```python
from build123d import *

# Parameters (mm, degrees)
BOX_W                  = 7.4
BOX_H                  = 7
BOX_DEPTH              = 0.2
BOX015_W               = 0.8
BOX015_H               = 9.4
BOX015_DEPTH           = 0.8
BOX015_PLACEMENT_ANGLE = 225
BOX014_W               = 0.4
BOX014_H               = 2.3
BOX014_DEPTH           = 1.91
BOX017_W               = 0.8
BOX017_H               = 9.4
BOX017_DEPTH           = 0.8
BOX017_PLACEMENT_ANGLE = 45
BOX013_W               = 0.4
BOX013_H               = 2.3
BOX013_DEPTH           = 1.91
BOX018_W               = 7.4
BOX018_H               = 9.4
BOX018_DEPTH           = 3.7
CYLINDER004_R          = 0.25
CYLINDER004_DEPTH      = 0.17
BOX024_W               = 0.9
BOX024_H               = 1.5
BOX024_DEPTH           = 0.15
FILLET006_R            = 0.2
CYLINDER006_R          = 0.25
CYLINDER006_DEPTH      = 0.17
BOX025_W               = 0.9
BOX025_H               = 1.5
BOX025_DEPTH           = 0.15
FILLET007_R            = 0.2
CYLINDER005_R          = 0.25
CYLINDER005_DEPTH      = 0.17
BOX026_W               = 0.9
BOX026_H               = 1.5
BOX026_DEPTH           = 0.15
FILLET008_R            = 0.2
CYLINDER007_R          = 0.25
CYLINDER007_DEPTH      = 0.17
BOX027_W               = 0.9
BOX027_H               = 1.5
BOX027_DEPTH           = 0.15
FILLET005_R            = 0.2
BOX023_W               = 0.8
BOX023_H               = 2.2
BOX023_DEPTH           = 0.8
BOX023_PLACEMENT_ANGLE = 45
BOX022_W               = 0.4
BOX022_H               = 2.2
BOX022_DEPTH           = 2
BOX020_W               = 0.8
BOX020_H               = 2.2
BOX020_DEPTH           = 0.8
BOX020_PLACEMENT_ANGLE = 45
BOX021_W               = 0.4
BOX021_H               = 2.2
BOX021_DEPTH           = 2
BOX019_W               = 7.7
BOX019_H               = 9.2
BOX019_DEPTH           = 4
FILLET009_R            = 0.2


with BuildPart() as cube:
    # Box → Box (new body)
    with BuildSketch(Plane(origin=(0.15, 2.2, -0.01), x_dir=(1, 0, 0), z_dir=(0, 0, 1))):
        with Locations((3.7, 3.5)):
            Rectangle(BOX_W, BOX_H)
    extrude(amount=BOX_DEPTH)


with BuildPart() as cube011:
    # Box015 → Box015 (new body)
    with BuildSketch(Plane.XY):
        with Locations((0.4, 4.7)):
            Rectangle(BOX015_W, BOX015_H)
    extrude(amount=BOX015_DEPTH)


with BuildPart() as cube011_1:
    # Box015 placement: moved
    add(cube011.part.moved(Location((7.4, -0.1, 2.06))).rotate(Axis((7.4, -0.1, 2.06), (0, 1, 0)), BOX015_PLACEMENT_ANGLE))


with BuildPart() as cut013:
    # Box014 → Box014 (new body)
    with BuildSketch(Plane(origin=(7, -0.1, 0.15), x_dir=(1, 0, 0), z_dir=(0, 0, 1))):
        with Locations((0.2, 1.15)):
            Rectangle(BOX014_W, BOX014_H)
    extrude(amount=BOX014_DEPTH)

    # Cut013: cut Cube011
    add(cube011_1.part, mode=Mode.SUBTRACT)


with BuildPart() as cut013_1:
    # Cut013 placement: moved
    add(cut013.part.moved(Location((0.15, 0, 0))))


with BuildPart() as cube013:
    # Box017 → Box017 (new body)
    with BuildSketch(Plane.XY):
        with Locations((0.4, 4.7)):
            Rectangle(BOX017_W, BOX017_H)
    extrude(amount=BOX017_DEPTH)


with BuildPart() as cube013_1:
    # Box017 placement: moved
    add(cube013.part.moved(Location((0.15, -0.1, 2.06))).rotate(Axis((0.15, -0.1, 2.06), (0, 1, 0)), BOX017_PLACEMENT_ANGLE))


with BuildPart() as cut022:
    # Box013 → Box013 (new body)
    with BuildSketch(Plane(origin=(0.15, -0.1, 0.15), x_dir=(1, 0, 0), z_dir=(0, 0, 1))):
        with Locations((0.2, 1.15)):
            Rectangle(BOX013_W, BOX013_H)
    extrude(amount=BOX013_DEPTH)

    # Cut022: cut Cube013
    add(cube013_1.part, mode=Mode.SUBTRACT)


with BuildPart() as cut024:
    # Box018 → Box018 (new body)
    with BuildSketch(Plane(origin=(0.15, -0.1, 0.15), x_dir=(1, 0, 0), z_dir=(0, 0, 1))):
        with Locations((3.7, 4.7)):
            Rectangle(BOX018_W, BOX018_H)
    extrude(amount=BOX018_DEPTH)

    # Cut023: cut Cut022
    add(cut022.part, mode=Mode.SUBTRACT)

    # Cut024: cut Cut013
    add(cut013_1.part, mode=Mode.SUBTRACT)


with BuildPart() as cylinder004:
    # Cylinder004 → Cylinder004 (new body)
    with BuildSketch(Plane(origin=(-0.9, 2.95, -0.01), x_dir=(1, 0, 0), z_dir=(0, 0, 1))):
        Circle(CYLINDER004_R)
    extrude(amount=CYLINDER004_DEPTH)


with BuildPart() as foot012:
    # Box024 → Box024 (new body)
    with BuildSketch(Plane(origin=(-0.9, 2.2, 0), x_dir=(1, 0, 0), z_dir=(0, 0, 1))):
        with Locations((0.45, 0.75)):
            Rectangle(BOX024_W, BOX024_H)
    extrude(amount=BOX024_DEPTH)

    # Cut021: cut Cylinder004
    add(cylinder004.part, mode=Mode.SUBTRACT)

    # Fillet006
    fillet006_edges = [foot012.edges().sort_by_distance(p)[0] for p in [
        (-0.9, 2.7, 0.075),
        (-0.9, 2.2, 0.075),
        (-0.9, 3.2, 0.075),
        (-0.9, 3.7, 0.075),
    ]]
    fillet(fillet006_edges, radius=FILLET006_R)


with BuildPart() as cylinder006:
    # Cylinder006 → Cylinder006 (new body)
    with BuildSketch(Plane(origin=(-0.9, 8.45, -0.01), x_dir=(1, 0, 0), z_dir=(0, 0, 1))):
        Circle(CYLINDER006_R)
    extrude(amount=CYLINDER006_DEPTH)


with BuildPart() as foot013:
    # Box025 → Box025 (new body)
    with BuildSketch(Plane(origin=(-0.9, 7.7, 0), x_dir=(1, 0, 0), z_dir=(0, 0, 1))):
        with Locations((0.45, 0.75)):
            Rectangle(BOX025_W, BOX025_H)
    extrude(amount=BOX025_DEPTH)

    # Cut016: cut Cylinder006
    add(cylinder006.part, mode=Mode.SUBTRACT)

    # Fillet007
    fillet007_edges = [foot013.edges().sort_by_distance(p)[0] for p in [
        (-0.9, 8.2, 0.075),
        (-0.9, 7.7, 0.075),
        (-0.9, 8.7, 0.075),
        (-0.9, 9.2, 0.075),
    ]]
    fillet(fillet007_edges, radius=FILLET007_R)


with BuildPart() as cylinder005:
    # Cylinder005 → Cylinder005 (new body)
    with BuildSketch(Plane(origin=(8.6, 2.95, -0.01), x_dir=(1, 0, 0), z_dir=(0, 0, 1))):
        Circle(CYLINDER005_R)
    extrude(amount=CYLINDER005_DEPTH)


with BuildPart() as foot014:
    # Box026 → Box026 (new body)
    with BuildSketch(Plane(origin=(7.7, 2.2, 0), x_dir=(1, 0, 0), z_dir=(0, 0, 1))):
        with Locations((0.45, 0.75)):
            Rectangle(BOX026_W, BOX026_H)
    extrude(amount=BOX026_DEPTH)

    # Cut014: cut Cylinder005
    add(cylinder005.part, mode=Mode.SUBTRACT)

    # Fillet008
    fillet008_edges = [foot014.edges().sort_by_distance(p)[0] for p in [
        (8.6, 2.2, 0.075),
        (8.6, 3.7, 0.075),
        (8.6, 2.7, 0.075),
        (8.6, 3.2, 0.075),
    ]]
    fillet(fillet008_edges, radius=FILLET008_R)


with BuildPart() as cylinder007:
    # Cylinder007 → Cylinder007 (new body)
    with BuildSketch(Plane(origin=(8.6, 8.45, -0.01), x_dir=(1, 0, 0), z_dir=(0, 0, 1))):
        Circle(CYLINDER007_R)
    extrude(amount=CYLINDER007_DEPTH)


with BuildPart() as foot009:
    # Box027 → Box027 (new body)
    with BuildSketch(Plane(origin=(7.7, 7.7, 0), x_dir=(1, 0, 0), z_dir=(0, 0, 1))):
        with Locations((0.45, 0.75)):
            Rectangle(BOX027_W, BOX027_H)
    extrude(amount=BOX027_DEPTH)

    # Cut015: cut Cylinder007
    add(cylinder007.part, mode=Mode.SUBTRACT)

    # Fillet005
    fillet005_edges = [foot009.edges().sort_by_distance(p)[0] for p in [
        (8.6, 7.7, 0.075),
        (8.6, 9.2, 0.075),
        (8.6, 8.2, 0.075),
        (8.6, 8.7, 0.075),
    ]]
    fillet(fillet005_edges, radius=FILLET005_R)


with BuildPart() as cube019:
    # Box023 → Box023 (new body)
    with BuildSketch(Plane.XY):
        with Locations((0.4, 1.1)):
            Rectangle(BOX023_W, BOX023_H)
    extrude(amount=BOX023_DEPTH)


with BuildPart() as cube019_1:
    # Box023 placement: moved
    add(cube019.part.moved(Location((0, 0, 2))).rotate(Axis((0, 0, 2), (0, 1, 0)), BOX023_PLACEMENT_ANGLE))


with BuildPart() as right_side_cutout001:
    # Box022 → Box022 (new body)
    with BuildSketch(Plane.XY):
        with Locations((0.2, 1.1)):
            Rectangle(BOX022_W, BOX022_H)
    extrude(amount=BOX022_DEPTH)

    # Cut018: cut Cube019
    add(cube019_1.part, mode=Mode.SUBTRACT)


with BuildPart() as right_side_cutout001_1:
    # Cut018 placement: moved
    add(right_side_cutout001.part.moved(Location((7.7, 0, 0))))


with BuildPart() as part_mirroring001:
    # Part__Mirroring001: instance of Right Side Cutout001
    add(right_side_cutout001_1.part.mirror(Plane(origin=(7.7, 0, 0), x_dir=(0, -1, 0), z_dir=(1, 0, 0))))


with BuildPart() as cube016:
    # Box020 → Box020 (new body)
    with BuildSketch(Plane.XY):
        with Locations((0.4, 1.1)):
            Rectangle(BOX020_W, BOX020_H)
    extrude(amount=BOX020_DEPTH)


with BuildPart() as cube016_1:
    # Box020 placement: moved
    add(cube016.part.moved(Location((0, 0, 2))).rotate(Axis((0, 0, 2), (0, 1, 0)), BOX020_PLACEMENT_ANGLE))


with BuildPart() as left_side_cutout001:
    # Box021 → Box021 (new body)
    with BuildSketch(Plane.XY):
        with Locations((0.2, 1.1)):
            Rectangle(BOX021_W, BOX021_H)
    extrude(amount=BOX021_DEPTH)

    # Cut020: cut Cube016
    add(cube016_1.part, mode=Mode.SUBTRACT)


with BuildPart() as metal_shell:
    # Box019 → Box019 (new body)
    with BuildSketch(Plane.XY):
        with Locations((3.85, 4.6)):
            Rectangle(BOX019_W, BOX019_H)
    extrude(amount=BOX019_DEPTH)

    # Cut019: cut Left Side Cutout001
    add(left_side_cutout001.part, mode=Mode.SUBTRACT)

    # Cut017: cut Part__Mirroring001
    add(part_mirroring001.part, mode=Mode.SUBTRACT)

    # Fillet009
    fillet009_edges = [metal_shell.edges().sort_by_distance(p)[0] for p in [
        (0, 4.6, 4),
        (7.7, 4.6, 4),
    ]]
    fillet(fillet009_edges, radius=FILLET009_R)

    # Fusion001: union Foot012, Foot013, Foot014, Foot009
    add(foot012.part)
    add(foot013.part)
    add(foot014.part)
    add(foot009.part)

    # Cut025: cut Cut024
    add(cut024.part, mode=Mode.SUBTRACT)

    # Cut: cut Cube
    add(cube.part, mode=Mode.SUBTRACT)


solid = metal_shell.part
```
Geometry: final body of the model. Coordinates: model frame, mm. Round coordinates to 2 decimals unless told otherwise and drop trailing zeros. Write each loop counter-clockwise with the first axis right and the second up, starting at its lowest first coordinate (ties: lowest second). Pieces come first, ordered by that corner, then holes. Notation, with made-up numbers: M -30.5,12.25 L -7.5,12.25 A9 cw -7.5,28.25 Z; hole C -29,75 d5. An arc over 180 degrees is marked long. Answer in a Markdown table with one row per item. Add a question column.
(1) Cut plane C-C, the plane z = 3.4. Return the cut outline in (x, y).
(2) Cut plane D-D, the plane y = 1.25. Return the cut outline in (x, z).
(3) Draft query along Z for faces 1 (the face through (0.55, 1, 1)), 2 (the face through (0.4, 1, 1)). Return one class per face: pulls with the +Z half, pulls with the -Z half, needs draft (parallel to the pull), parting line crosses it, or undercut.
(4) Ray query, L1, parallel to X at y = 1, z = 0.95. Return the intervals inside material, ascending.
(5) Contact query for flat-ended pins moving along their axis: pin 1 (1 mm diameter, centred on y = 6, z = 3.5, fed in from -X); pin 2 (0.7 mm diameter, centred on x = 8.5, y = 2.5, fed in from +Z); pin 3 (1 mm diameter, centred on x = 1, z = 1, fed in from +Y); pin 4 (0.7 mm diameter, centred on x = -0.5, z = 1.5, fed in from -Y). Output: stop coordinate, or through.
(6) Cut plane A-A, the plane z = 0.8. Return the cut outline in (x, y), then the cut area to 3 significant figures.
(7) Cut plane B-B, the plane x = 6.25. Return the cut outline in (y, z), then the cut area to 3 significant figures.
Established:
| question | item | result |
|---|---|---|
| 1 | outline | M 0,0 L 0.15,0 L 0.15,9.2 L 0,9.2 Z; M 7.55,0 L 7.7,0 L 7.7,9.2 L 7.55,9.2 Z |
| 2 | outline | M 0,2 L 0.4,1.6 L 0.4,0 L 7.3,0 L 7.3,1.6 L 7.7,2 L 7.7,3.8 A0.2 ccw 7.5,4 L 0.2,4 A0.2 ccw 0,3.8 Z; hole M 0.15,2.06 L 0.55,1.66 L 0.55,0.15 L 7.15,0.15 L 7.15,1.66 L 7.55,2.06 L 7.55,3.85 L 0.15,3.85 Z |
| 3 | face 1 | undercut |
| 3 | face 2 | needs draft |
| 4 | L1 | 0.4 to 0.55, 7.15 to 7.3 |
| 5 | pin 1 | x = 0 |
| 5 | pin 2 | z = 0.15 |
| 5 | pin 3 | y = 2.2 |
| 5 | pin 4 | through |
| 6 | outline | M 0,2.2 L 0.15,2.2 L 0.15,9.2 L 0,9.2 Z; M 0.4,0 L 0.55,0 L 0.55,2.2 L 0.4,2.2 Z; M 7.15,0 L 7.3,0 L 7.3,2.2 L 7.15,2.2 Z; M 7.55,2.2 L 7.7,2.2 L 7.7,9.2 L 7.55,9.2 Z |
| 6 | area | 2.76 mm² |
| 7 | outline | M 0,0 L 2.2,0 L 2.2,0.15 L 0,0.15 Z; M 0,3.85 L 9.2,3.85 L 9.2,4 L 0,4 Z |
| 7 | area | 1.71 mm² |
